Input: part model. Units: mm. Frame: model coordinates. Face numbers are marked on the shaded views. A direction names the side the tool comes from. Coordinates: 2 decimals unless noted, no trailing zeros. Loops run counter-clockwise (first coordinate to the right, second up) from the corner with the lowest first, then second, coordinate; pieces in that order, holes last. Notation, with made-up numbers: (86, 43) -> (123, 43) arc R13 ccw to (123, 66) -> close; hole circle Ø9 at (-30, -12.5). An arc over 180 degrees is marked (long way). Put each result on its own line as item: value. Start each with the question number.
1) Contact query for flat-ended pins moving along their axis: P1, Ø1.3, axis at y = 3, z = 2.5, coming from the -X side; P2, Ø2.5, axis at x = 9, y = 1.5, coming from the +Z side; P3, Ø1.5, axis at y = 6, z = 1.5, coming from the -X side; P4, Ø3, axis at x = -18.5, y = 7, coming from the +Z side. Output: stop coordinate, or through.
2) Cut plane B-B (z = -1.9). State how many separate pieces and enclosed holes the cut face has, plus the area to 3 significant figures.
3) Pull-direction query (Y, two-part tool) for the marked faces 1, 2, 3 and 4; classes: pulls with the +Y half, pulls with the -Y half, needs draft (parallel to the pull), parting line crosses it, or undercut.
4) Material intervals for L1, parallel to Y at x = 0, z = 2.1 (3 decimals); L2, parallel to X at y = 4.5, z = -0.9; L3, parallel to X at y = 6.5, z = 1.9, sorted ascending.
5) Set-up query: the marked faces 5, 6, 7 and 8. Return all of +Z, -Z, +X, -X, +Y, -Y with unobstructed straight access to the full face (end or side cutting, diameter ignored); none if empty.
6) Cut plane D-D (x = 8.5). Return the cut outline in (y, z), plus the area to 3 significant figures.
from build123d import *

# Parameters (mm, degrees)
SKETCH1_W           = 38.1
SKETCH1_H           = 2.159
BOSS_EXTRUDE1_DEPTH = 8.255
CUT_EXTRUDE1_DEPTH  = 12.7
FILLET5_R           = 0.4826
FILLET7_R           = 0.4445
SKETCH3_W           = 4.953
SKETCH3_H           = 8.255
BOSS_EXTRUDE2_DEPTH = 1.27
CUT_EXTRUDE4_DEPTH  = 5.699
FILLET9_R           = 0.6985
SKETCH4_R           = 5.11953367
BOSS_EXTRUDE3_DEPTH = 4.699
CUT_EXTRUDE3_DEPTH  = 4.699
BOSS_EXTRUDE4_DEPTH = 0.889
SKETCH10_W          = 8.28565978
SKETCH10_H          = 8.255
BOSS_EXTRUDE5_DEPTH = 0.762
FILLET10_R          = 0.4445
SKETCH11_R          = 1.27
CUT_EXTRUDE5_DEPTH  = 1.762


with BuildPart() as part:
    # Sketch1 → Boss-Extrude1 (new body)
    with BuildSketch(Plane(origin=(0, 0, 0), x_dir=(1, 0, 0), z_dir=(0, 1, 0))):
        Rectangle(SKETCH1_W, SKETCH1_H)
    extrude(amount=BOSS_EXTRUDE1_DEPTH)

    # Sketch2 → Cut-Extrude1 (cut)
    with BuildSketch(Plane.XY.offset(1.0795)):
        with BuildLine():
            Line((0.435059279, 1.422786249), (14.097, 3.048))
            ThreePointArc((14.097, 3.048), (15.901602081, 5.08), (14.097, 7.112))
            Line((14.097, 7.112), (14.839370062, 13.352542684))
            Line((14.839370062, 13.352542684), (0.435059279, 13.41059889))
            Line((0.435059279, 13.41059889), (-0.435059279, 13.41059889))
            Line((-0.435059279, 13.41059889), (0, 8.763))
            ThreePointArc((0, 8.763), (-3.676547786, 5.297911397), (-0.435059279, 1.422786249))
            ThreePointArc((-0.435059279, 1.422786249), (0, 1.397), (0.435059279, 1.422786249))
        make_face()
    extrude(amount=-CUT_EXTRUDE1_DEPTH, mode=Mode.SUBTRACT)

    # Fillet5
    fillet5_edges = [part.edges().sort_by_distance(p)[0] for p in [
        (14.232970383, 8.255, 0),
        (14.097, 7.112, 0),
    ]]
    fillet(fillet5_edges, radius=FILLET5_R)

    # Fillet7
    fillet7_edges = [part.edges().sort_by_distance(p)[0] for p in [
        (-1.866511184, 8.255, 0),
    ]]
    fillet(fillet7_edges, radius=FILLET7_R)

    # Sketch3 → Boss-Extrude2 (add)
    with BuildSketch(Plane.XY.offset(1.0795)):
        with Locations((16.5735, 4.1275)):
            Rectangle(SKETCH3_W, SKETCH3_H)
    boss_extrude2 = extrude(amount=BOSS_EXTRUDE2_DEPTH)

    # Mirror2: Boss-Extrude2 across plane
    add(boss_extrude2.mirror(Plane.XY))

    # Sketch8 → Cut-Extrude4 (cut, through all)
    with BuildSketch(Plane.XY.offset(2.3495)):
        Polygon((15.3035, 1.6891), (17.8435, 1.6891), (17.228717877, 0), (15.918282123, 0), align=None)
    extrude(amount=-CUT_EXTRUDE4_DEPTH, mode=Mode.SUBTRACT)

    # Fillet9
    fillet9_edges = [part.edges().sort_by_distance(p)[0] for p in [
        (14.097, 0, -1.7145),
        (14.097, 0, 1.7145),
        (14.097, 8.255, -1.7145),
        (19.05, 0, 0),
        (19.05, 8.255, 0),
    ]]
    fillet(fillet9_edges, radius=FILLET9_R)

    # Sketch4 → Boss-Extrude3 (add)
    with BuildSketch(Plane.XY.offset(2.3495)):
        with Locations((-18.415, 5.08)):
            Circle(SKETCH4_R)
        Polygon((-18.415, 0.589871939), (-22.905128061, 5.08), (-18.415, 9.570128061), (-13.924871939, 5.08), align=None, mode=Mode.SUBTRACT)
    extrude(amount=-BOSS_EXTRUDE3_DEPTH)

    # Sketch7 → Cut-Extrude3 (cut)
    with BuildSketch(Plane.XY.offset(2.3495)):
        Polygon((-22.905128061, 5.08), (-18.415, 9.570128061), (-13.924871939, 5.08), (-18.415, 0.589871939), align=None)
    extrude(amount=-CUT_EXTRUDE3_DEPTH, mode=Mode.SUBTRACT)

    # Sketch9 → Boss-Extrude4 (add)
    with BuildSketch(Plane.XY.offset(1.0795)):
        with BuildLine():
            Line((-3.095258632, 8.255), (-5.000258632, 8.255))
            Line((-5.000258632, 8.255), (-5.000258632, 0))
            Line((-5.000258632, 0), (0.110401148, 0))
            Line((0.110401148, 0), (3.285401148, 0))
            Line((3.285401148, 0), (3.285401148, 1.761860681))
            Line((3.285401148, 1.761860681), (0.435059279, 1.422786249))
            ThreePointArc((0.435059279, 1.422786249), (-3.261402544, 3.368935289), (-2.761923087, 7.516446154))
            ThreePointArc((-2.761923087, 7.516446154), (-2.690112248, 7.993356932), (-3.095258632, 8.255))
        make_face()
    extrude(amount=BOSS_EXTRUDE4_DEPTH)

    # Sketch10 → Boss-Extrude5 (add)
    with BuildSketch(Plane.XY.offset(1.9685)):
        with Locations((-0.857428742, 4.1275)):
            Rectangle(SKETCH10_W, SKETCH10_H)
    extrude(amount=BOSS_EXTRUDE5_DEPTH)

    # Fillet10
    fillet10_edges = [part.edges().sort_by_distance(p)[0] for p in [
        (-5.000258632, 8.255, 1.905),
        (3.285401148, 8.255, 2.3495),
    ]]
    fillet(fillet10_edges, radius=FILLET10_R)

    # Sketch11 → Cut-Extrude5 (cut, through all)
    with BuildSketch(Plane(origin=(0, 0, 1.9685), x_dir=(-1, 0, 0), z_dir=(0, 0, -1))):
        with Locations((0, 5.08)):
            Circle(SKETCH11_R)
    extrude(amount=-CUT_EXTRUDE5_DEPTH, mode=Mode.SUBTRACT)


solid = part.part
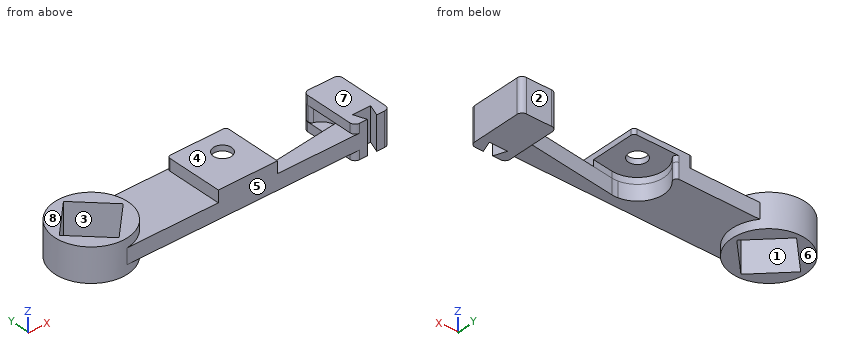
Results found:
1. P1: stops at x = -23.33
1. P2: stops at z = 1.08
1. P3: stops at x = -23.53
1. P4: passes through
2. separate pieces: 2
2. enclosed holes: 1
2. area: 79.2 mm2
3. face 1: undercut
3. face 2: pulls with the +Y half
3. face 3: undercut
3. face 4: needs draft
4. L1: y = 0 to 3.81, 6.35 to 8.255
4. L2: x = -23.5 to -22.33, -14.5 to -3.64, 15.82 to 19.05
4. L3: x = -23.33 to -21.49, -15.34 to -13.5, -5 to -3.4, 14.1 to 19.05
5. face 5: +Z, -Z, +X, -Y
5. face 6: -Z, +X, -X, +Y, -Y
5. face 7: +Z, +X, +Y, -Y
5. face 8: +Z, -X, +Y, -Y
6. outline: (0, -1.08) -> (2.38, -1.08) -> (2.38, 1.08) -> (0, 1.08) -> close
6. area: 5.14 mm2
